Could you check a few things on this drawing? It's one solid part, dimensions in mm from its lowest x, y, z. A direction names the side the tool comes from. Give positions to 0.01 mm unless a question says otherwise; leave off trailing zeros. Loops run counter-clockwise (first coordinate to the right, second up) from the corner with the lowest first, then second, coordinate; pieces in that order, holes last. Notation, with made-up numbers: (81.25, 41.5) - (134.25, 41.5) arc R22 cw to (134.25, 80.5) - close; hole circle Ø2 at (73, 43). An arc over 180 degrees is marked (long way). Write each question's results on one line, items separated by ' | '. Start each with the question number.
(1) For pin 1 (6.5 mm diameter, centred on x = 19.85, y = 36.27, fed in from +Z), with a flat end and sliding along its axis, tell me the tip position at first contact or that it passes through.
(2) Suppose I cut it at B-B (x = 61.5). Please give me the cut outline in (y, z), and give its area (3 significant figures).
(3) Suppose I cut it at C-C (x = 12). Please give me the cut outline in (y, z), and give its area (3 significant figures).
(4) Suppose I cut it at A-A (z = 18.5). Please give me the cut outline in (x, y), and give its area (3 significant figures).
(5) I need wall thicknesses on line 1 (Y direction, x = 74, z = 15); line 2 (X direction, y = 81, z = 2.5); line 3 (Y direction, x = 75, z = 3.45). Which ranges of each line are inside material? Lowest first, please.
(6) On a 3-axis mill with a long thin cutter (end or side, diameter ignored), from which of +Z, -Z, +X, -X, +Y, -Y can I reach the whole of each face in a straight line? I mean the marked faces 5 and 6. Say none if no direction works.
(7) If we mould it in two halves opening along Y, with no side actions, what happens to the marked faces 1, 2, 3 and 4? For each: released by +Y, released by -Y, zero draft, split by the parting line, or undercut.
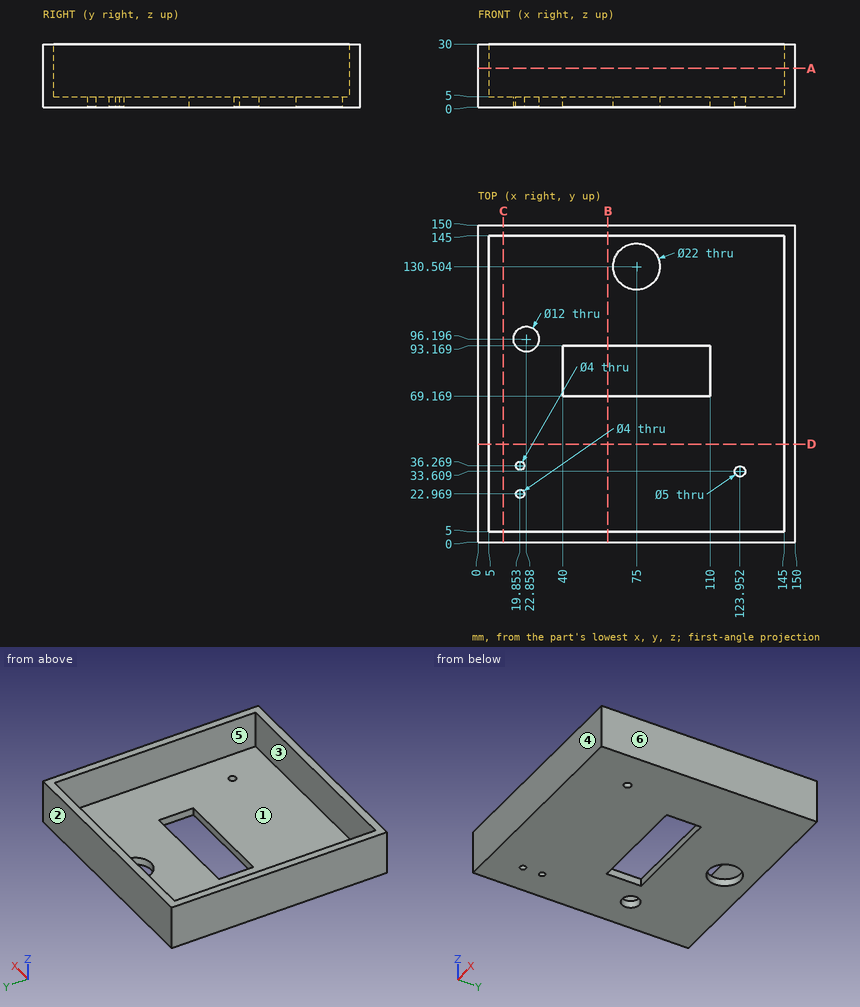
Output values:
1) pin 1: z = 5
2) outline: (0, 0) - (69.17, 0) - (69.17, 5) - (5, 5) - (5, 30) - (0, 30) - close; (93.17, 0) - (150, 0) - (150, 30) - (145, 30) - (145, 5) - (93.17, 5) - close | area: 880 mm2
3) outline: (0, 0) - (150, 0) - (150, 30) - (145, 30) - (145, 5) - (5, 5) - (5, 30) - (0, 30) - close | area: 1,000 mm2
4) outline: (0, 0) - (150, 0) - (150, 150) - (0, 150) - close; hole (5, 5) - (145, 5) - (145, 145) - (5, 145) - close | area: 2,900 mm2
5) line 1: 0 to 5, 145 to 150 | line 2: 0 to 40, 110 to 150 | line 3: 0 to 69.17, 93.17 to 119.5, 141.5 to 150
6) face 5: +Z | face 6: +Z, -Z, +X, +Y, -Y
7) face 1: undercut | face 2: released by +Y | face 3: undercut | face 4: released by -Y
